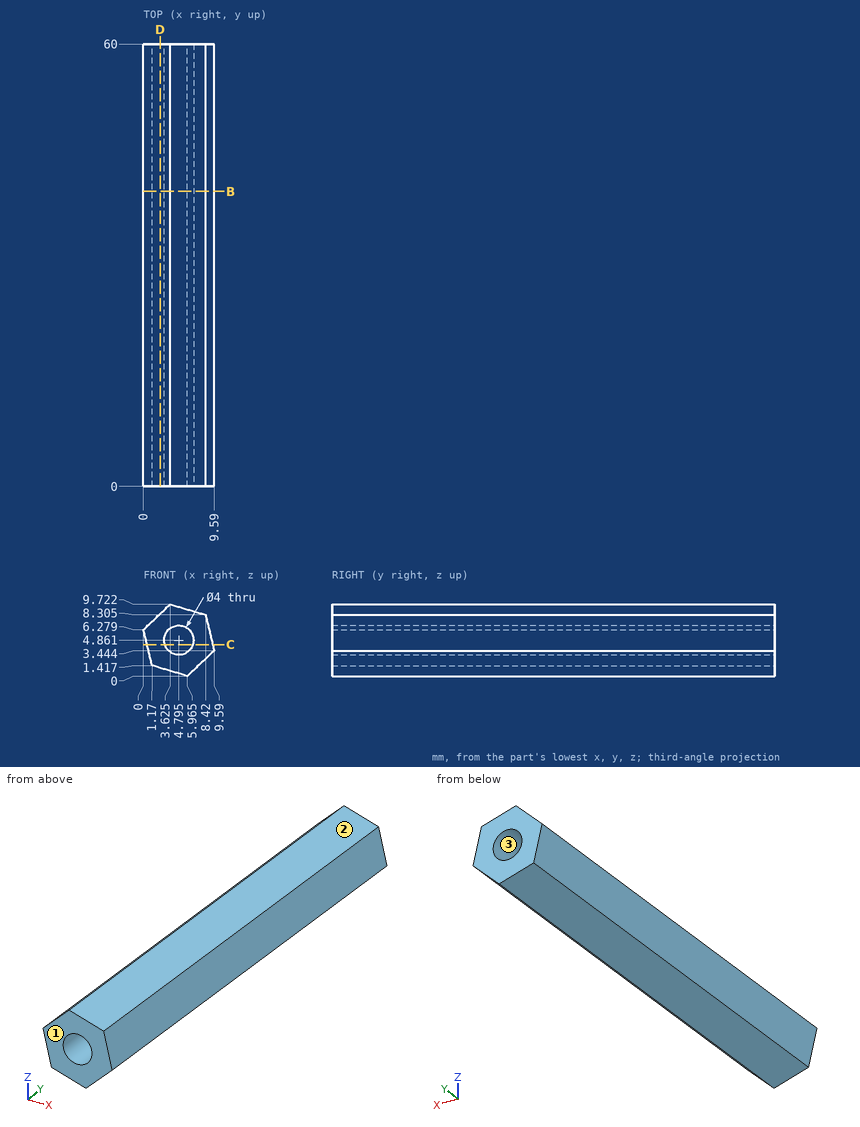
Geometry: see drawing. Coordinates: mm, zero at the bounding-box minimum. Give positions to 0.01 mm unless a question says otherwise; leave off trailing zeros. Loops run counter-clockwise (first coordinate to the right, second up) from the corner with the lowest first, then second, coordinate; pieces in that order, holes last. Notation, with made-up numbers: (50.25, 32) -> (74.25, 32) arc R11 ccw to (74.25, 38) -> close; hole circle Ø11 at (-25, 89.5). An arc over 180 degrees is marked (long way). Use one line per item in the form item = value.
Item 1: Section query B-B on y = 40. Output: boundary loops of the cut face in (x, z) (1 decimal).
A:
outline = (0, 6.3) -> (1.2, 1.4) -> (6, 0) -> (9.6, 3.4) -> (8.4, 8.3) -> (3.6, 9.7) -> close; hole circle Ø4 at (4.8, 4.9)
Item 2: Draft query along Z for the marked faces 1, 2 and 3. Return one class per face: pulls with the +Z half, pulls with the -Z half, needs draft (parallel to the pull), parting line crosses it, or undercut.
A:
face_1 = needs draft
face_2 = pulls with the +Z half
face_3 = undercut
Item 3: Line query: probe 1 along Z at (x, y) = (3, 54) (1 decimal); probe 2 along Z at (x, y) = (4.5, 10) (1 decimal); probe 3 along X at (y, z) = (14, 3.75) (1 decimal). Output: solid intervals per line, ascending.
A:
probe_1 = 0.9 to 4, 5.7 to 9.1
probe_2 = 0.4 to 2.9, 6.8 to 9.5
probe_3 = 0.6 to 3.1, 6.5 to 9.5
Item 4: Section query C-C on z = 4.25. Output: boundary loops of the cut face in (x, y) (1 decimal), and give its area (3 significant figures).
A:
outline = (0.5, 0) -> (2.9, 0) -> (2.9, 60) -> (0.5, 60) -> close; (6.7, 0) -> (9.4, 0) -> (9.4, 60) -> (6.7, 60) -> close
area = 306 mm^2
Item 5: Pin query (flat end, axial travel): P1, Ø2, axis at x = 3, y = 14, coming from the -Z side; P2, Ø2, axis at x = 8.5, y = 19.5, coming from the -Z side; P3, Ø1, axis at x = 1, y = 31.5, coming from the +Z side (1 decimal). Return the tip coordinate at first contact, or that it passes through.
A:
P1 = 0.58
P2 = 1.46
P3 = 7.7
Item 6: Section query D-D on x = 2.25. Output: boundary loops of the cut face in (y, z).
A:
outline = (0, 1.1) -> (60, 1.1) -> (60, 8.42) -> (0, 8.42) -> close
